Model file for the job. Use its own axes, mm. A direction names the side the tool comes from. Coordinates: 2 decimals unless noted, no trailing zeros. Loops run counter-clockwise (first coordinate to the right, second up) from the corner with the lowest first, then second, coordinate; pieces in that order, holes last.
from build123d import *

# Parameters (mm, degrees)
F2_R     = 38.1
F3_DEPTH = 12.7
F1_R     = 38.1
F4_DEPTH = 12.7
F0_R     = 22.446656
F5_DEPTH = 12.7


with BuildPart() as f3:
    # F2 (on Right) → F3 (new body, symmetric)
    with BuildSketch(Plane.YZ):
        Circle(F2_R)
    extrude(amount=F3_DEPTH, both=True)

    # F1 (on Front) → F4 (join, symmetric)
    with BuildSketch(Plane.XZ):
        Circle(F1_R)
    extrude(amount=F4_DEPTH, both=True)

    # F0 (on Top) → F5 (join, symmetric)
    with BuildSketch(Plane.XY):
        Circle(F0_R)
    extrude(amount=F5_DEPTH, both=True)


solid = f3.part
Q1. Drill centre lines: line 1 (Y direction, x = 16, z = -21.5); line 2 (X direction, y = -3, z = 23.5). Where is each one in solid material? Low to high.
Answers:
line 1: y = -12.7 to 12.7
line 2: x = -29.99 to 29.99
Q2. Which spindle directions (+Z, -Z, +X, -X, +Y, -Y) get a long thin tool onto all of the face, cutting with end or side? Do faces 1 (the cylindrical face through (-7.7, -0.2, -38.1)), 2 (the flat face through (15, -15, -12.7)), 3 (the flat face through (15, 15, -12.7)), 4 (the flat face through (12.7, 0, -37)), 5 (the flat face through (0, -12.7, 37)). Say none if no direction does.
Answers:
face 1: -Z, -X
face 2: -Z, +X, -Y
face 3: -Z, +X, +Y
face 4: -Z, +X, +Y, -Y
face 5: +Z, +X, -X, -Y
Q3. Slice it at B-B (x = -5.5). List the corners of the cut face in (y, z).
Answers:
outline: (-12.7, -37.7) - (-5.5, -37.7) arc R38.1 ccw to (5.5, -37.7) - (12.7, -37.7) - (12.7, -35.92) arc R38.1 ccw to (12.7, 35.92) - (12.7, 37.7) - (5.5, 37.7) arc R38.1 ccw to (-5.5, 37.7) - (-12.7, 37.7) - (-12.7, 35.92) arc R38.1 ccw to (-12.7, -35.92) - close
Q4. Flat gauge pins, fed straight in: P1, Ø1.1, axis at y = -1, z = 37, coming from the -X side; P2, Ø12.5, axis at y = 26, z = -5, coming from the +X side; P3, Ø12.5, axis at x = -19.5, z = 8.5, coming from the +Y side. Where does each tip first touch, or does it go through?
Answers:
P1: stops at x = -12.7
P2: stops at x = 12.7
P3: stops at y = 18.12
Q5. Slice it at D-D (z = 11.5). List the corners of the cut face in (x, y).
Answers:
outline: (-36.32, -12.7) - (-18.51, -12.7) arc R22.45 ccw to (-12.7, -18.51) - (-12.7, -36.32) - (12.7, -36.32) - (12.7, -18.51) arc R22.45 ccw to (18.51, -12.7) - (36.32, -12.7) - (36.32, 12.7) - (18.51, 12.7) arc R22.45 ccw to (12.7, 18.51) - (12.7, 36.32) - (-12.7, 36.32) - (-12.7, 18.51) arc R22.45 ccw to (-18.51, 12.7) - (-36.32, 12.7) - close
Q6. Slice it at C-C (y = 6.5). List the corners of the cut face in (x, z), and give its area (3 significant figures).
Answers:
outline: (-12.7, -37.54) - (-6.5, -37.54) arc R38.1 ccw to (6.5, -37.54) - (12.7, -37.54) - (12.7, -35.92) arc R38.1 ccw to (12.7, 35.92) - (12.7, 37.54) - (6.5, 37.54) arc R38.1 ccw to (-6.5, 37.54) - (-12.7, 37.54) - (-12.7, 35.92) arc R38.1 ccw to (-12.7, -35.92) - close
area: 4,580 mm2
Q7. Slice it at A-A (z = 1.5). List the corners of the cut face in (x, y), and give its area (3 significant figures).
Answers:
outline: (-38.07, -12.7) - (-18.51, -12.7) arc R22.45 ccw to (-12.7, -18.51) - (-12.7, -38.07) - (12.7, -38.07) - (12.7, -18.51) arc R22.45 ccw to (18.51, -12.7) - (38.07, -12.7) - (38.07, 12.7) - (18.51, 12.7) arc R22.45 ccw to (12.7, 18.51) - (12.7, 38.07) - (-12.7, 38.07) - (-12.7, 18.51) arc R22.45 ccw to (-18.51, 12.7) - (-38.07, 12.7) - close
area: 3,300 mm2
